For this review, take the finished solid that the model builds, in its own axes (mm). A direction names the side the tool comes from. Round coordinates to 2 decimals unless told otherwise and drop trailing zeros. Write each loop counter-clockwise with the first axis right and the second up, starting at its lowest first coordinate (ties: lowest second). Pieces come first, ordered by that corner, then holes. Notation, with made-up numbers: (78.5, 83) - (125.5, 83) arc R29 cw to (125.5, 108) - close; hole circle Ø7 at (-36.75, -27). An arc over 180 degrees is marked (long way). One line per item, written item: value. Start each with the question number.
Q1. Add section B-B on x = -18. Write out the cut boundary in (y, z), and give its area (3 significant figures).
Q2. Add section C-C on z = 25.5. Write out the cut boundary in (x, y), and give its area (3 significant figures).
Q3. Tool access review of faces 1 (the face through (-10, 2, 45)), 2 (the face through (-12.55, 8.92, 57.32)), 3 (the face through (29.756, 2.574, 4.93)), 4 (the face through (-33.244, -4.426, 4.93)), 5 (the face through (11, -5, 45)): name each direction out of +Z, -Z, +X, -X, +Y, -Y from which nothing blocks a thin tool from reaching the whole face with its end or side.
Q4. Mouldability with a two-part tool opening along Y and no side actions: class faces 6 (the face through (-0.362, 3.215, 4.93)), 7 (the face through (15.756, -11.426, 27.255)), 8 (the face through (-9, 16, 45)) as +Y half, -Y half, draft (parallel to the pull), parting line (faces both ways), or undercut.
Q5. Add section A-A on y = 20. Write out the cut boundary in (x, z).
Q6. Clearance check with flat-ended pins moving along their axes: pin 1 Ø4 at (y, z) = (-13, 11.5) entering from +X; pin 2 Ø8 at (x, z) = (-24, 44.5) entering from -Y; pin 3 Ø10 at (y, z) = (18, 47) entering from +X; pin 4 Ø8 at (x, y) = (-2.75, 16.46) entering from +Z. State where each tip first meets the part, or that it passes through.
Q7. For probe 1 along Z at (x, y) = (-35.5, 20); probe 2 along X at (y, z) = (16.5, 31); probe 3 along Z at (x, y) = (-39, 33), list the stretches that pass through material, from the lowest coordinate up.
Q8. Add section D-D on x = -45. Write out the cut boundary in (y, z), and give its area (3 significant figures).
```python
from build123d import *

# Parameters (mm, degrees)
F0_W     = 75
F0_H     = 45
F0_R     = 2.5
F1_DEPTH = 10
F2_DEPTH = 45
F3_R     = 19.69693
F4_DEPTH = 25


with BuildPart() as f1:
    # F0 (on Top) → F1 (new body)
    with BuildSketch(Plane.XY):
        Rectangle(F0_W, F0_H)
        with Locations((-30.746223, -11.535893)):
            Circle(F0_R, mode=Mode.SUBTRACT)
        with Locations((-23.746223, -11.535893)):
            Circle(F0_R, mode=Mode.SUBTRACT)
        with Locations((-16.746223, -11.535893)):
            Circle(F0_R, mode=Mode.SUBTRACT)
        with Locations((-9.746223, -11.535893)):
            Circle(F0_R, mode=Mode.SUBTRACT)
        with Locations((-2.746223, -11.535893)):
            Circle(F0_R, mode=Mode.SUBTRACT)
        with Locations((-30.746223, -4.535893)):
            Circle(F0_R, mode=Mode.SUBTRACT)
        with Locations((-23.746223, -4.535893)):
            Circle(F0_R, mode=Mode.SUBTRACT)
        with Locations((-16.746223, -4.535893)):
            Circle(F0_R, mode=Mode.SUBTRACT)
        with Locations((-9.746223, -4.535893)):
            Circle(F0_R, mode=Mode.SUBTRACT)
        with Locations((-2.746223, -4.535893)):
            Circle(F0_R, mode=Mode.SUBTRACT)
        with Locations((4.253777, -11.535893)):
            Circle(F0_R, mode=Mode.SUBTRACT)
        with Locations((11.253777, -11.535893)):
            Circle(F0_R, mode=Mode.SUBTRACT)
        with Locations((18.253777, -11.535893)):
            Circle(F0_R, mode=Mode.SUBTRACT)
        with Locations((25.253777, -11.535893)):
            Circle(F0_R, mode=Mode.SUBTRACT)
        with Locations((32.253777, -11.535893)):
            Circle(F0_R, mode=Mode.SUBTRACT)
        with Locations((4.253777, -4.535893)):
            Circle(F0_R, mode=Mode.SUBTRACT)
        with Locations((11.253777, -4.535893)):
            Circle(F0_R, mode=Mode.SUBTRACT)
        with Locations((18.253777, -4.535893)):
            Circle(F0_R, mode=Mode.SUBTRACT)
        with Locations((25.253777, -4.535893)):
            Circle(F0_R, mode=Mode.SUBTRACT)
        with Locations((32.253777, -4.535893)):
            Circle(F0_R, mode=Mode.SUBTRACT)
        with Locations((-30.746223, 2.464107)):
            Circle(F0_R, mode=Mode.SUBTRACT)
        with Locations((-23.746223, 2.464107)):
            Circle(F0_R, mode=Mode.SUBTRACT)
        with Locations((-30.746223, 9.464107)):
            Circle(F0_R, mode=Mode.SUBTRACT)
        with Locations((-23.746223, 9.464107)):
            Circle(F0_R, mode=Mode.SUBTRACT)
        with Locations((-16.746223, 2.464107)):
            Circle(F0_R, mode=Mode.SUBTRACT)
        with Locations((-9.746223, 2.464107)):
            Circle(F0_R, mode=Mode.SUBTRACT)
        with Locations((-2.746223, 2.464107)):
            Circle(F0_R, mode=Mode.SUBTRACT)
        with Locations((-16.746223, 9.464107)):
            Circle(F0_R, mode=Mode.SUBTRACT)
        with Locations((-9.746223, 9.464107)):
            Circle(F0_R, mode=Mode.SUBTRACT)
        with Locations((-2.746223, 9.464107)):
            Circle(F0_R, mode=Mode.SUBTRACT)
        with Locations((-30.746223, 16.464107)):
            Circle(F0_R, mode=Mode.SUBTRACT)
        with Locations((-23.746223, 16.464107)):
            Circle(F0_R, mode=Mode.SUBTRACT)
        with Locations((-16.746223, 16.464107)):
            Circle(F0_R, mode=Mode.SUBTRACT)
        with Locations((-9.746223, 16.464107)):
            Circle(F0_R, mode=Mode.SUBTRACT)
        with Locations((-2.746223, 16.464107)):
            Circle(F0_R, mode=Mode.SUBTRACT)
        with Locations((4.253777, 2.464107)):
            Circle(F0_R, mode=Mode.SUBTRACT)
        with Locations((11.253777, 2.464107)):
            Circle(F0_R, mode=Mode.SUBTRACT)
        with Locations((18.253777, 2.464107)):
            Circle(F0_R, mode=Mode.SUBTRACT)
        with Locations((4.253777, 9.464107)):
            Circle(F0_R, mode=Mode.SUBTRACT)
        with Locations((11.253777, 9.464107)):
            Circle(F0_R, mode=Mode.SUBTRACT)
        with Locations((18.253777, 9.464107)):
            Circle(F0_R, mode=Mode.SUBTRACT)
        with Locations((25.253777, 2.464107)):
            Circle(F0_R, mode=Mode.SUBTRACT)
        with Locations((32.253777, 2.464107)):
            Circle(F0_R, mode=Mode.SUBTRACT)
        with Locations((25.253777, 9.464107)):
            Circle(F0_R, mode=Mode.SUBTRACT)
        with Locations((32.253777, 9.464107)):
            Circle(F0_R, mode=Mode.SUBTRACT)
        with Locations((4.253777, 16.464107)):
            Circle(F0_R, mode=Mode.SUBTRACT)
        with Locations((11.253777, 16.464107)):
            Circle(F0_R, mode=Mode.SUBTRACT)
        with Locations((18.253777, 16.464107)):
            Circle(F0_R, mode=Mode.SUBTRACT)
        with Locations((25.253777, 16.464107)):
            Circle(F0_R, mode=Mode.SUBTRACT)
        with Locations((32.253777, 16.464107)):
            Circle(F0_R, mode=Mode.SUBTRACT)
        with Locations((-23.746223, 16.464107)):
            Circle(F0_R)
        with Locations((-23.746223, 9.464107)):
            Circle(F0_R)
        with Locations((-23.746223, 2.464107)):
            Circle(F0_R)
        with Locations((-23.746223, -4.535893)):
            Circle(F0_R)
        with Locations((-16.746223, -4.535893)):
            Circle(F0_R)
        with Locations((-9.746223, -4.535893)):
            Circle(F0_R)
        with Locations((-2.746223, -4.535893)):
            Circle(F0_R)
        with Locations((-2.746223, -11.535893)):
            Circle(F0_R)
        with Locations((4.253777, -4.535893)):
            Circle(F0_R)
        with Locations((11.253777, 2.464107)):
            Circle(F0_R)
        with Locations((18.253777, 9.464107)):
            Circle(F0_R)
        with Locations((25.253777, 16.464107)):
            Circle(F0_R)
    extrude(amount=F1_DEPTH)

    # F0 (on Top) → F2 (join)
    with BuildSketch(Plane.XY):
        with Locations((-30.746223, 16.464107)):
            Circle(F0_R)
        with Locations((-9.746223, 16.464107)):
            Circle(F0_R)
        with Locations((-9.746223, 2.464107)):
            Circle(F0_R)
        with Locations((11.253777, -4.535893)):
            Circle(F0_R)
        with Locations((25.253777, -4.535893)):
            Circle(F0_R)
        with Locations((18.253777, -11.535893)):
            Circle(F0_R)
    extrude(amount=F2_DEPTH)

    # F3 (on face) → F4 (join)
    with BuildSketch(Plane.XY.offset(45)):
        with Locations((-30.746223, 16.464107)):
            Circle(F3_R)
    extrude(amount=F4_DEPTH)


solid = f1.part
```
Result set:
1. outline: (-22.5, 0) - (-13.7, 0) - (-13.7, 10) - (-22.5, 10) - close; (-9.37, 0) - (0.3, 0) - (0.3, 10) - (-9.37, 10) - close; (1.45, 45) - (31.48, 45) - (31.48, 70) - (1.45, 70) - close; (4.63, 0) - (7.3, 0) - (7.3, 10) - (4.63, 10) - close; (11.63, 0) - (14.3, 0) - (14.3, 10) - (11.63, 10) - close; (18.63, 0) - (22.5, 0) - (22.5, 10) - (18.63, 10) - close
1. area: 1,030 mm^2
2. outline: circle Ø5 at (-30.75, 16.46); circle Ø5 at (-9.75, 2.46); circle Ø5 at (-9.75, 16.46); circle Ø5 at (11.25, -4.54); circle Ø5 at (18.25, -11.54); circle Ø5 at (25.25, -4.54)
2. area: 118 mm^2
3. face 1: +Z, +X, -Y
3. face 2: +Z
3. face 3: +Z, -Z
3. face 4: -Z
3. face 5: +Z, +X, +Y, -Y
4. face 6: undercut
4. face 7: parting line
4. face 8: draft
5. outline: (-50.12, 45) - (-11.37, 45) - (-11.37, 70) - (-50.12, 70) - close; (-37.5, 0) - (37.5, 0) - (37.5, 10) - (-37.5, 10) - close
6. pin 1: stops at x = 37.5
6. pin 2: stops at y = -3.04
6. pin 3: stops at x = -7.25
6. pin 4: stops at z = 10
7. probe 1: z = 0 to 10, 45 to 70
7. probe 2: x = -33.25 to -28.25, -12.25 to -7.25
7. probe 3: z = 45 to 70
8. outline: (2.87, 45) - (30.06, 45) - (30.06, 70) - (2.87, 70) - close
8. area: 680 mm^2
